Read the model definition and answer for the solid it produces. Units are mm, in the model's axes. A direction names the side the tool comes from. Coordinates: 2 decimals unless noted, no trailing zeros. Write each loop counter-clockwise with the first axis right and the second up, starting at its lowest first coordinate (ties: lowest second). Pieces come first, ordered by that corner, then holes.
1) The part is cut by section B-B (z = 11.5). Determine the outline of the cut face in (x, y), then the cut area to 3 significant figures.
2) Which of the six approach directions +Z, -Z, +X, -X, +Y, -Y give full straight-line access (tool end or side, diameter ignored) to faces 1 (the face through (-1.38, -6.2, 0.63)), 2 (the face through (1.5, 0.07, -2.96))?
3) Each of these flat-tipped pins is pushed along its axis until it touches: pin 1 Ø1.5 at (x, z) = (-1, -2.5) entering from +Y; pin 2 Ø4 at (y, z) = (2.5, 9) entering from -X; pin 3 Ø2 at (x, z) = (1, -0.5) entering from -Y. Where does it stop, or does it pass through?
4) The part is cut by section A-A (z = 5). Determine the outline of the cut face in (x, y).
5) Find the intervals of material crossed by line 1 (X direction, y = -0.25, z = 5); line 2 (X direction, y = -4, z = 0.5); line 3 (Y direction, x = 3.25, z = 3), in increasing order.
from build123d import *

# Parameters (mm, degrees)
SKETCH1_R           = 6.35
BOSS_EXTRUDE1_DEPTH = 1.27
SKETCH3_R           = 1.5
BOSS_EXTRUDE2_DEPTH = 6


# Read off the part's stored shape, not the designer's step: Loft1
with BuildPart() as part:
    # Sketch1 → Boss-Extrude1 (new body)
    with BuildSketch(Plane.XY):
        Circle(SKETCH1_R)
    extrude(amount=BOSS_EXTRUDE1_DEPTH)

    # Loft1 outline → Loft1 (revolve)
    with BuildSketch(Plane.XZ):
        Polygon((6.35, 1.27), (0, 25.4), (0, 1.27), align=None)
    revolve(axis=Axis((0, 0, 0), (0, 0, 1)))

    # Sketch3 → Boss-Extrude2 (add)
    with BuildSketch(Plane(origin=(0, 0, 0), x_dir=(-1, 0, 0), z_dir=(0, 0, -1))):
        Circle(SKETCH3_R)
    extrude(amount=BOSS_EXTRUDE2_DEPTH)


solid = part.part
Reported:
1. outline: circle Ø7.32 at (0, 0)
1. area: 42.0 mm2
2. face 1: +Z, -Z
2. face 2: -Z
3. pin 1: stops at y = 1.48
3. pin 2: stops at x = -4.56
3. pin 3: stops at y = -6.35
4. outline: circle Ø10.74 at (0, 0)
5. line 1: x = -5.36 to 5.36
5. line 2: x = -4.93 to 4.93
5. line 3: y = -4.92 to 4.92
